Source: CAD feature listing. Evaluate the final solid. Frame: model axes, mm. Face numbers are marked on the shaded views. A direction names the side the tool comes from. Round coordinates to 2 decimals unless told otherwise and drop trailing zeros. Write each loop counter-clockwise with the first axis right and the second up, starting at its lowest first coordinate (ties: lowest second). Pieces come first, ordered by that corner, then holes. Notation, with made-up numbers: M 85.25,-6.5 L 102.25,-6.5 A21 ccw 102.25,5.5 Z; hole C 33,-35.5 d11. An arc over 180 degrees is marked long. Use a Markdown table: item, result.
```python
from build123d import *

# Parameters (mm, degrees)
MAIN_SHELL_SKETCH_W     = 11.5
MAIN_SHELL_SKETCH_H     = 4
MAIN_SHELL_DEPTH        = 20
CONNECTOR_HOLE_SKETCH_W = 2
CONNECTOR_HOLE_SKETCH_H = 2.5
CONNECTOR_HOLES_DEPTH   = 5.5


with BuildPart() as part:
    # Main_shell_sketch → Main_shell (new body)
    with BuildSketch(Plane(origin=(0, 0, 0), x_dir=(0, 0, -1), z_dir=(1, 0, 0))):
        with BuildLine():
            Line((-6, 2), (-6, -2))
            ThreePointArc((-6, -2), (-5.926776695, -2.176776695), (-5.75, -2.25))
            Line((-5.75, -2.25), (5.75, -2.25))
            ThreePointArc((5.75, -2.25), (5.926776695, -2.176776695), (6, -2))
            Line((6, -2), (6, 2))
            ThreePointArc((6, 2), (5.926776695, 2.176776695), (5.75, 2.25))
            Line((5.75, 2.25), (-5.75, 2.25))
            ThreePointArc((-5.75, 2.25), (-5.926776695, 2.176776695), (-6, 2))
        make_face()
        Rectangle(MAIN_SHELL_SKETCH_W, MAIN_SHELL_SKETCH_H, mode=Mode.SUBTRACT)
    extrude(amount=-MAIN_SHELL_DEPTH)

    # Connector_hole_sketch → Connector_holes (cut, through all)
    with BuildSketch(Plane(origin=(0, 2.25, 0), x_dir=(1, 0, 0), z_dir=(0, 1, 0))):
        with Locations((-6, 2.75)):
            Rectangle(CONNECTOR_HOLE_SKETCH_W, CONNECTOR_HOLE_SKETCH_H)
        with Locations((-6, -2.75)):
            Rectangle(CONNECTOR_HOLE_SKETCH_W, CONNECTOR_HOLE_SKETCH_H)
        with BuildLine():
            Line((-18, -1.5), (-18, 1.5))
            ThreePointArc((-18, 1.5), (-17.5, 2), (-17, 1.5))
            Line((-17, 1.5), (-17, -1.5))
            ThreePointArc((-17, -1.5), (-17.5, -2), (-18, -1.5))
        make_face()
    extrude(amount=-CONNECTOR_HOLES_DEPTH, mode=Mode.SUBTRACT)


solid = part.part
```
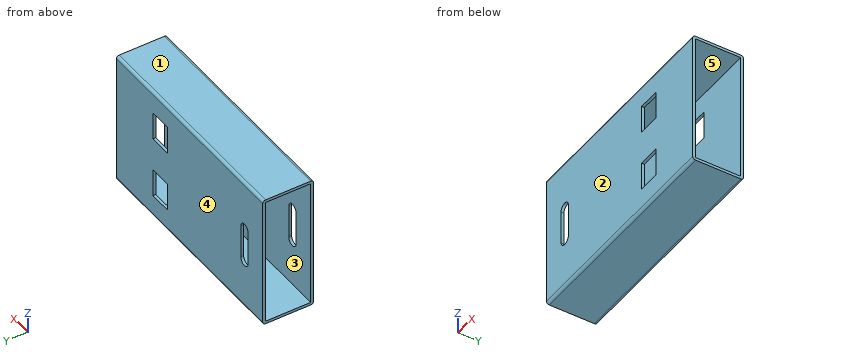
Q1. Reachability of the marked faces 4 and 5 from +Z, -Z, +X, -X, +Y, -Y: full face, straight path, thin tool, end or side. Return the list, or none.
Results are:
| item | result |
|---|---|
| face 4 | +Z, -Z, +X, -X, +Y |
| face 5 | +X, -X |
Q2. Section D-D on y = 1.7. Return loops of the section in (x, z), plus the area to 3 significant figures.
Results are:
| item | result |
|---|---|
| outline | M -20,-6 L 0,-6 L 0,-5.75 L -20,-5.75 Z; M -20,5.75 L 0,5.75 L 0,6 L -20,6 Z |
| area | 10.0 mm^2 |
Q3. Section C-C on x = -13.75. Return loops of the section in (y, z).
Results are:
| item | result |
|---|---|
| outline | M -2.25,-5.75 A0.25 ccw -2,-6 L 2,-6 A0.25 ccw 2.25,-5.75 L 2.25,5.75 A0.25 ccw 2,6 L -2,6 A0.25 ccw -2.25,5.75 Z; hole M -2,-5.75 L 2,-5.75 L 2,5.75 L -2,5.75 Z |
Q4. Section B-B on z = 2.75. Return loops of the section in (x, y).
Results are:
| item | result |
|---|---|
| outline | M -20,-2.25 L -7,-2.25 L -7,-2 L -20,-2 Z; M -20,2 L -7,2 L -7,2.25 L -20,2.25 Z; M -5,-2.25 L 0,-2.25 L 0,-2 L -5,-2 Z; M -5,2 L 0,2 L 0,2.25 L -5,2.25 Z |
Q5. Mould query, pull axis Y, two halves, no side actions, for the marked faces 1, 2 and 3. Classes: +Y half, -Y half, draft (parallel to the pull), parting line (faces both ways), or undercut.
Results are:
| item | result |
|---|---|
| face 1 | draft |
| face 2 | -Y half |
| face 3 | undercut |
Q6. Line query: L1, parallel to Y at x = -15, z = -4.75; L2, parallel to Z at x = -15.5, y = -1.5. Output: solid intervals per line, ascending.
Results are:
| item | result |
|---|---|
| L1 | -2.25 to -2, 2 to 2.25 |
| L2 | -6 to -5.75, 5.75 to 6 |
Q7. Section A-A on x = -17.5. Return loops of the section in (y, z), plus the area to 3 significant figures.
Results are:
| item | result |
|---|---|
| outline | M -2.25,-5.75 A0.25 ccw -2,-6 L 2,-6 A0.25 ccw 2.25,-5.75 L 2.25,-2 L 2,-2 L 2,-5.75 L -2,-5.75 L -2,-2 L -2.25,-2 Z; M -2.25,2 L -2,2 L -2,5.75 L 2,5.75 L 2,2 L 2.25,2 L 2.25,5.75 A0.25 ccw 2,6 L -2,6 A0.25 ccw -2.25,5.75 Z |
| area | 5.95 mm^2 |
